from build123d import *

# Parameters (mm, degrees)
SALIENTE_EXTRUIR1_DEPTH      = 3
SALIENTE_EXTRUIR1_2_DEPTH    = 3
SALIENTE_EXTRUIR2_DEPTH      = 1
SALIENTE_EXTRUIR2_DEPTH_BACK = 1
CROQUIS3_W                   = 5
CROQUIS3_H                   = 5
SALIENTE_EXTRUIR3_DEPTH      = 120
SALIENTE_EXTRUIR4_DEPTH      = 1
SALIENTE_EXTRUIR4_DEPTH_BACK = 1
CROQUIS7_W                   = 5
CROQUIS7_H                   = 5
SALIENTE_EXTRUIR6_DEPTH      = 120
CROQUIS8_W                   = 85
CROQUIS8_H                   = 17
SALIENTE_EXTRUIR7_DEPTH      = 5
CROQUIS9_W                   = 16
CROQUIS9_H                   = 4
CORTAR_EXTRUIR1_DEPTH        = 70
CROQUIS10_W                  = 30.5
CROQUIS10_H                  = 15.5
CORTAR_EXTRUIR2_DEPTH        = 2


with BuildPart() as part:
    # Croquis1 → Saliente-Extruir1 (new body)
    with BuildSketch(Plane(origin=(0, 0, 0), x_dir=(1, 0, 0), z_dir=(0, 1, 0))):
        with BuildLine():
            Line((-6.5, -7.5), (6.5, -7.5))
            ThreePointArc((6.5, -7.5), (7.207106781, -7.207106781), (7.5, -6.5))
            Line((7.5, -6.5), (7.5, 6.5))
            ThreePointArc((7.5, 6.5), (7.207106781, 7.207106781), (6.5, 7.5))
            Line((6.5, 7.5), (-6.5, 7.5))
            ThreePointArc((-6.5, 7.5), (-7.207106781, 7.207106781), (-7.5, 6.5))
            Line((-7.5, 6.5), (-7.5, -6.5))
            ThreePointArc((-7.5, -6.5), (-7.207106781, -7.207106781), (-6.5, -7.5))
        make_face()
    extrude(amount=SALIENTE_EXTRUIR1_DEPTH)

    # Croquis2 → Saliente-Extruir2 (add, two sides: drawn at the far end of the back side and taken through both)
    with BuildSketch(Plane(origin=(0, 0, 0), x_dir=(0, 0, -1), z_dir=(1, 0, 0)).offset(-SALIENTE_EXTRUIR2_DEPTH_BACK)):
        Polygon((-7.5, 3), (-2.5, 8), (-2.5, 3), align=None)
        Polygon((2.5, 3), (7.5, 3), (2.5, 8), align=None)
    extrude(amount=SALIENTE_EXTRUIR2_DEPTH + SALIENTE_EXTRUIR2_DEPTH_BACK)

    # Croquis3 → Saliente-Extruir3 (add)
    with BuildSketch(Plane(origin=(0, 3, 0), x_dir=(1, 0, 0), z_dir=(0, 1, 0))):
        Rectangle(CROQUIS3_W, CROQUIS3_H)
    extrude(amount=SALIENTE_EXTRUIR3_DEPTH)



with BuildPart() as body_2:
    # Croquis1 → Saliente-Extruir1 2 (new body)
    with BuildSketch(Plane(origin=(0, 0, 0), x_dir=(1, 0, 0), z_dir=(0, 1, 0))):
        with BuildLine():
            Line((77.5, -6.5), (77.5, 6.5))
            ThreePointArc((77.5, 6.5), (77.792893219, 7.207106781), (78.5, 7.5))
            Line((78.5, 7.5), (91.5, 7.5))
            ThreePointArc((91.5, 7.5), (92.207106781, 7.207106781), (92.5, 6.5))
            Line((92.5, 6.5), (92.5, -6.5))
            ThreePointArc((92.5, -6.5), (92.207106781, -7.207106781), (91.5, -7.5))
            Line((91.5, -7.5), (78.5, -7.5))
            ThreePointArc((78.5, -7.5), (77.792893219, -7.207106781), (77.5, -6.5))
        make_face()
    extrude(amount=SALIENTE_EXTRUIR1_2_DEPTH)

    # Croquis5 → Saliente-Extruir4 (add, two sides: drawn at the far end of the back side and taken through both)
    with BuildSketch(Plane(origin=(85, 0, 0), x_dir=(0, 0, -1), z_dir=(1, 0, 0)).offset(-SALIENTE_EXTRUIR4_DEPTH_BACK)):
        Polygon((-7.5, 3), (-2.5, 8), (-2.5, 3), align=None)
        Polygon((2.5, 8), (2.5, 3), (7.5, 3), align=None)
    extrude(amount=SALIENTE_EXTRUIR4_DEPTH + SALIENTE_EXTRUIR4_DEPTH_BACK)

    # Croquis7 → Saliente-Extruir6 (add)
    with BuildSketch(Plane(origin=(0, 3, 0), x_dir=(1, 0, 0), z_dir=(0, 1, 0))):
        with Locations((85, 0)):
            Rectangle(CROQUIS7_W, CROQUIS7_H)
    extrude(amount=SALIENTE_EXTRUIR6_DEPTH)


with BuildPart() as part_1:
    add(part.part)

    add(body_2.part)  # Saliente-Extruir7 merges body 2
    # Croquis8 → Saliente-Extruir7 (add)
    with BuildSketch(Plane(origin=(0, 118, 0), x_dir=(1, 0, 0), z_dir=(0, 1, 0))):
        with Locations((42.5, 0)):
            Rectangle(CROQUIS8_W, CROQUIS8_H)
    extrude(amount=SALIENTE_EXTRUIR7_DEPTH)

    # Croquis9 → Cortar-Extruir1 (cut)
    with BuildSketch(Plane.ZY.offset(2.5)):
        with Locations((0, 121)):
            Rectangle(CROQUIS9_W, CROQUIS9_H)
    extrude(amount=-CORTAR_EXTRUIR1_DEPTH, mode=Mode.SUBTRACT)

    # Croquis10 → Cortar-Extruir2 (cut)
    with BuildSketch(Plane.XZ.offset(-118)):
        with Locations((42.5, 0)):
            Rectangle(CROQUIS10_W, CROQUIS10_H)
    extrude(amount=-CORTAR_EXTRUIR2_DEPTH, mode=Mode.SUBTRACT)


solid = part_1.part
Model file for the job. Use its own axes, mm. A direction names the side the tool comes from. Give positions to 0.01 mm unless a question says otherwise; leave off trailing zeros. Order: outer loops, then holes, each group sorted by start corner. A loop starts at its lowest first (then second) coordinate and runs counter-clockwise, first axis right, second up. Notation, with made-up numbers: (79, -23) - (87, -23) arc R17 ccw to (87, -19) - close; hole circle Ø5 at (-14, 31.25). An arc over 180 degrees is marked (long way). Write item = value, one per line. Start each with the question number.
1. Which spindle directions (+Z, -Z, +X, -X, +Y, -Y) get a long thin tool onto all of the face, cutting with end or side? Do faces 1 (the flat face through (1, 4, -4)), 2 (the flat face through (82.5, 60, 0)), 3 (the flat face through (0, 1, -7.5)), 4 (the flat face through (-2.5, 60, 0)), 5 (the flat face through (-1, 4, -4)). Say none if no direction does.
2. Cut at C-C, the plane x = 4.5. List the corners of the cut face in (y, z).
3. Probe line 1 along Y through (x, z) = (3.5, 0.25); line 2 along X through (y, z) = (69, -0.5); line 3 along Y through (x, z) = (18, -4.75). List the from-to ranges inside material, lowest first.
4. Drop flat-ended pins along their axis: P1, Ø1, axis at y = 90, z = -0.5, coming from the -X side; P2, Ø4, axis at x = 0, y = 71.5, coming from the -Z side; P3, Ø5, axis at x = 36, z = -4, coming from the -Y side; P4, Ø6, axis at y = 62, z = -2, coming from the +X side. Give the stop position or say it passes through.
5. Two-plate mould, pull along X, no slides. Class faces 6 (the flat face through (33, 121, -8)), 7 (the flat face through (86, 4, -4)), 8 (the flat face through (7.5, 1, 0)), 9 (the flat face through (2.5, 60, 0)): pulls with the +X half, pulls with the -X half, needs draft (parallel to the pull), parting line crosses it, or undercut.
6. Cut at A-A, the plane z = -0.75. List the corners of the cut face in (x, y), and give its area (3 significant figures).
7. Cut at D-D, the plane x = 39. List the corners of the cut face in (y, z), and give its area (3 significant figures).
8. Cut at B-B, the plane y = 90. List the corners of the cut face in (x, z).
Taken from the geometry:
q1.face_1 = -Z
q1.face_2 = +Z, -Z
q1.face_3 = -Z, +X, -X, -Y
q1.face_4 = +Z, -Z, -X, +Y
q1.face_5 = -Z, -X, +Y
q2.outline = (0, -7.5) - (3, -7.5) - (3, 7.5) - (0, 7.5) - close; (118, -8.5) - (123, -8.5) - (123, -8) - (119, -8) - (119, 8) - (123, 8) - (123, 8.5) - (118, 8.5) - close
q3.line_1 = 0 to 3, 118 to 119
q3.line_2 = -2.5 to 2.5, 82.5 to 87.5
q3.line_3 = 118 to 119
q4.P1 = -2.5
q4.P2 = -2.5
q4.P3 = through
q4.P4 = 87.5
q5.face_6 = needs draft
q5.face_7 = pulls with the +X half
q5.face_8 = undercut
q5.face_9 = undercut
q6.outline = (-7.5, 0) - (7.5, 0) - (7.5, 3) - (2.5, 3) - (2.5, 118) - (27.25, 118) - (27.25, 119) - (-2.5, 119) - (-2.5, 3) - (-7.5, 3) - close; (57.75, 118) - (82.5, 118) - (82.5, 3) - (77.5, 3) - (77.5, 0) - (92.5, 0) - (92.5, 3) - (87.5, 3) - (87.5, 123) - (67.5, 123) - (67.5, 119) - (57.75, 119) - close
q6.area = 1,380 mm²
q7.outline = (118, -8.5) - (123, -8.5) - (123, -8) - (119, -8) - (119, -7.75) - (118, -7.75) - close; (118, 7.75) - (119, 7.75) - (119, 8) - (123, 8) - (123, 8.5) - (118, 8.5) - close
q7.area = 5.50 mm²
q8.outline = (-2.5, -2.5) - (2.5, -2.5) - (2.5, 2.5) - (-2.5, 2.5) - close; (82.5, -2.5) - (87.5, -2.5) - (87.5, 2.5) - (82.5, 2.5) - close
